```python
from build123d import *

# Parameters (mm, degrees)
F0_R     = 75
F0_R_2   = 20.666788
F1_DEPTH = 25
F2_R     = 22.5
F3_DEPTH = 25.001
F4_R     = 71.929289
F4_R_2   = 68.929292
F5_DEPTH = 15


with BuildPart() as f1:
    # F0 (on Front) → F1 (new body)
    with BuildSketch(Plane.XZ):
        Circle(F0_R)
        Circle(F0_R_2, mode=Mode.SUBTRACT)
        Circle(F0_R_2)
    extrude(amount=F1_DEPTH)

    # F2 (on face) → F3 (cut, through all)
    with BuildSketch(Plane.XZ.offset(25)):
        Circle(F2_R)
    extrude(amount=-F3_DEPTH, mode=Mode.SUBTRACT)

    # F4 (on face) → F5 (cut)
    with BuildSketch(Plane.XZ.offset(25)):
        Circle(F4_R)
        Circle(F4_R_2, mode=Mode.SUBTRACT)
    extrude(amount=-F5_DEPTH, mode=Mode.SUBTRACT)


solid = f1.part
```
Geometry: final body of the model. Coordinates: model frame, mm. A direction names the side the tool comes from. Round coordinates to 2 decimals unless told otherwise and drop trailing zeros. Order: outer loops, then holes, each group sorted by start corner. A loop starts at its lowest first (then second) coordinate and runs counter-clockwise, first axis right, second up. Notation, with made-up numbers: M 12.5,-37 L 46.5,-37 A10 ccw 46.5,-30 Z; hole C 22,2.5 d6. An arc over 180 degrees is marked long. Use one line per item in the form item = value. Start each with the question number.
Q1. Access query for faces 1 (the face through (5, -10, -69)), 2 (the face through (61, -25, -39)). Directions: +Z, -Z, +X, -X, +Y, -Y. A direction counts if a zero-diameter tool reaches every point of the face in a straight line with its end or side. Return the directions, or none.
Q2. Cut plane D-D (x = 58.5). Return loops of the section in (y, z), and give its area (3 significant figures).
Q3. Material intervals for line 1 (Z direction, x = 0, y = -13.5); line 2 (Z direction, x = 13.5, y = -14) (3 decimals); line 3 (X direction, y = -11.5, z = 11.5), sorted ascending. Write a range as [from, to].
Q4. Mould query, pull axis Z, two halves, no side actions, for faces 3 (the face through (-15.59, -17.6, -70.22)), 4 (the face through (-9.764, -12.325, 74.362)), 5 (the face through (-16.3, -25, 16.3)). Classes: +Z half, -Z half, draft (parallel to the pull), parting line (faces both ways), or undercut.
Q5. Cut plane C-C (y = -16.25). Return loops of the section in (x, z).
Q6. Cut plane A-A (x = 0). Return loops of the section in (y, z).
Q7. Pin query (flat end, axial travel): pin 1 Ø1.5 at (x, z) = (27.5, -58.5) entering from +Y; pin 2 Ø1 at (x, y) = (0.5, -8) entering from +Z; pin 3 Ø6 at (x, y) = (1, -22.5) entering from -Z; pin 4 Ø2 at (y, z) = (-17, -59.5) entering from -X. Return the tip coordinate at first contact, or that it passes through.
Q8. Cut plane B-B (z = 0). Return loops of the section in (x, y), and give its area (4 significant figures).
Geometry results:
q1.face_1 = -Y
q1.face_2 = +Z, -Z, +X, -X, -Y
q2.outline = M -25,-46.93 L 0,-46.93 L 0,46.93 L -25,46.93 L -25,41.85 L -10,41.85 L -10,36.46 L -25,36.46 L -25,-36.46 L -10,-36.46 L -10,-41.85 L -25,-41.85 Z
q2.area = 2,180 mm^2
q3.line_1 = [-75, -71.93], [-68.93, -22.5], [22.5, 68.93], [71.93, 75]
q3.line_2 = [-73.775, -70.651], [-67.594, -18], [18, 67.594], [70.651, 73.775]
q3.line_3 = [-74.11, -71], [-67.96, -19.34], [19.34, 67.96], [71, 74.11]
q4.face_3 = undercut
q4.face_4 = parting line
q4.face_5 = draft
q5.outline = C 0,0 d150; C 0,0 d137.86; hole C 0,0 d143.86; hole C 0,0 d45
q6.outline = M -25,-75 L 0,-75 L 0,-22.5 L -25,-22.5 L -25,-68.93 L -10,-68.93 L -10,-71.93 L -25,-71.93 Z; M -25,22.5 L 0,22.5 L 0,75 L -25,75 L -25,71.93 L -10,71.93 L -10,68.93 L -25,68.93 Z
q7.pin_1 = 0
q7.pin_2 = 75
q7.pin_3 = -75
q7.pin_4 = -46.93
q8.outline = M -75,-25 L -71.93,-25 L -71.93,-10 L -68.93,-10 L -68.93,-25 L -22.5,-25 L -22.5,0 L -75,0 Z; M 22.5,-25 L 68.93,-25 L 68.93,-10 L 71.93,-10 L 71.93,-25 L 75,-25 L 75,0 L 22.5,0 Z
q8.area = 2,535 mm^2
